The model under review builds one solid part; all positions refer to its coordinate system, in mm. A direction names the side the tool comes from. Coordinates: 2 decimals unless noted, no trailing zeros. One line per item, written item: value.
```python
from build123d import *

# Parameters (mm, degrees)
SKETCH_1_W          = 124
SKETCH_1_H          = 80
EXTRUDE_1_DEPTH     = 5
SKETCH_2_R          = 1.15
CUT_EXTRUDE_1_DEPTH = 74.952687578
SKETCH_2_3_R        = 1.75
CUT_EXTRUDE_2_DEPTH = 3


with BuildPart() as part:
    # Sketch 1 → Extrude 1 (new body)
    with BuildSketch(Plane(origin=(0, 0, 0), x_dir=(1, 0, 0), z_dir=(0, 1, 0))):
        Rectangle(SKETCH_1_W, SKETCH_1_H)
    extrude(amount=EXTRUDE_1_DEPTH)

    # Sketch 2 → Cut-Extrude 1 (cut, through all)
    with BuildSketch(Plane(origin=(0, 5, 0), x_dir=(1, 0, 0), z_dir=(0, 1, 0))):
        with Locations(Location((-57.5, 37.5, 0), (0, 0, 270))):
            Circle(SKETCH_2_R)
        with Locations(Location((-57.5, 17, 0), (0, 0, 270))):
            Circle(SKETCH_2_R)
        with Locations(Location((-57.5, -17, 0), (0, 0, 270))):
            Circle(SKETCH_2_R)
        with Locations(Location((-57.5, -37.5, 0), (0, 0, 270))):
            Circle(SKETCH_2_R)
        with Locations(Location((57.5, 37.5, 0), (0, 0, 270))):
            Circle(SKETCH_2_R)
        with Locations(Location((57.5, 17, 0), (0, 0, 270))):
            Circle(SKETCH_2_R)
        with Locations(Location((57.5, -17, 0), (0, 0, 270))):
            Circle(SKETCH_2_R)
        with Locations(Location((57.5, -37.5, 0), (0, 0, 270))):
            Circle(SKETCH_2_R)
    extrude(amount=-CUT_EXTRUDE_1_DEPTH, mode=Mode.SUBTRACT)

    # Sketch 2_3 → Cut-Extrude 2 (cut)
    with BuildSketch(Plane(origin=(0, 5, 0), x_dir=(1, 0, 0), z_dir=(0, 1, 0))):
        with Locations(Location((-57.5, 37.5, 0), (0, 0, 270))):
            Circle(SKETCH_2_3_R)
        with Locations(Location((-57.5, 17, 0), (0, 0, 270))):
            Circle(SKETCH_2_3_R)
        with Locations(Location((-57.5, -17, 0), (0, 0, 270))):
            Circle(SKETCH_2_3_R)
        with Locations(Location((-57.5, -37.5, 0), (0, 0, 270))):
            Circle(SKETCH_2_3_R)
        with Locations(Location((57.5, 37.5, 0), (0, 0, 270))):
            Circle(SKETCH_2_3_R)
        with Locations(Location((57.5, 17, 0), (0, 0, 270))):
            Circle(SKETCH_2_3_R)
        with Locations(Location((57.5, -17, 0), (0, 0, 270))):
            Circle(SKETCH_2_3_R)
        with Locations(Location((57.5, -37.5, 0), (0, 0, 270))):
            Circle(SKETCH_2_3_R)
    extrude(amount=-CUT_EXTRUDE_2_DEPTH, mode=Mode.SUBTRACT)


solid = part.part
```
(1) To check wall thickness, follow L1, parallel to X at y = 1, z = 17; L2, parallel to X at y = 3.1, z = 17. State the ranges of each line that lie inside material, in increasing order. Write a range as [from, to].
Checks:
L1: [-62, -58.65], [-56.35, 56.35], [58.65, 62]
L2: [-62, -59.25], [-55.75, 55.75], [59.25, 62]
(2) Insertion check: pin 1 Ø1 at (x, z) = (-58, -36.5) entering from +Y; pin 2 Ø2 at (x, z) = (57.5, 37.5) entering from -Y. Each pin has a flat end and moves straight along its axis. Give the tip position at first contact, or say it passes through.
Checks:
pin 1: y = 2
pin 2: through
(3) Tool access review of faces 1 (the face through (56.83, 3.521, -35.883)), 2 (the face through (-56.36, 1.01, -17.15)): name each direction out of +Z, -Z, +X, -X, +Y, -Y from which nothing blocks a thin tool from reaching the whole face with its end or side.
Checks:
face 1: +Y
face 2: +Y, -Y
(4) Draft analysis for pull direction Z (two halves, no side actions). For faces 3 (the face through (-1, 2, 40)), 4 (the face through (-1, 2, -40)), 5 (the face through (-1, 5, -1)), 6 (the face through (-58.17, 3.521, -35.883)), state which applies: pulls with the +Z half, pulls with the -Z half, needs draft (parallel to the pull), parting line crosses it, or undercut.
Checks:
face 3: pulls with the +Z half
face 4: pulls with the -Z half
face 5: needs draft
face 6: undercut
